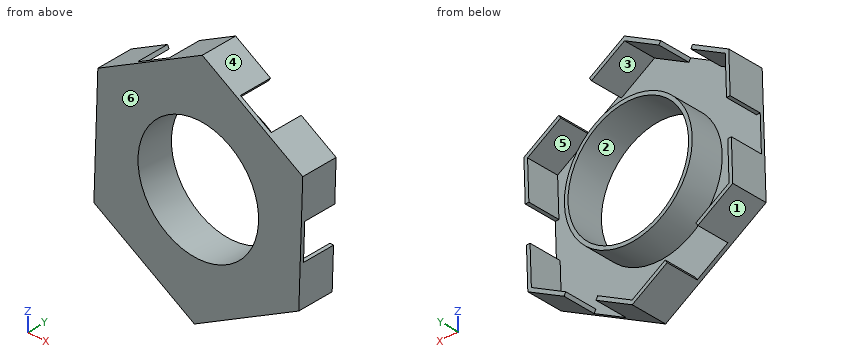
from build123d import *

# Parameters (mm, degrees)
SKETCH2_R           = 50
BOSS_EXTRUDE1_DEPTH = 30
SHELL1_T            = -3
CUT_EXTRUDE1_DEPTH  = 27


with BuildPart() as part:
    # Sketch2 → Boss-Extrude1 (new body)
    with BuildSketch(Plane(origin=(0, 0, 0), x_dir=(1, 0, 0), z_dir=(0, 1, 0))):
        Polygon((-83.314894361, -51.8841181), (3.275517147, -98.09487408), (86.590411508, -46.21075598), (83.314894361, 51.8841181), (-3.275517147, 98.09487408), (-86.590411508, 46.21075598), align=None)
        with Locations(Location((0, 0, 0), (0, 0, 270))):
            Circle(SKETCH2_R, mode=Mode.SUBTRACT)
    extrude(amount=BOSS_EXTRUDE1_DEPTH)

    # Shell1
    shell1_openings = [part.faces().sort_by_distance(p)[0] for p in [
        (-38.787596874, 30, 72.680784017),
    ]]
    offset(amount=SHELL1_T, openings=shell1_openings, kind=Kind.INTERSECTION)

    # Sketch8 → Cut-Extrude1 (cut)
    with BuildSketch(Plane(origin=(0, 30, 0), x_dir=(1, 0, 0), z_dir=(0, 1, 0))):
        Polygon((53.253129093, 67.9271981), (51.840669496, 65.280510003), (25.373788523, 79.405105982), (26.786248121, 82.051794079), align=None)
        Polygon((84.452062159, 17.828325695), (85.453243709, -12.154963576), (82.454914782, -12.255081731), (81.453733232, 17.72820754), align=None)
        Polygon((57.665814038, -64.223468384), (32.200114616, -80.082161676), (30.614245287, -77.535591734), (56.079944709, -61.676898442), align=None)
        Polygon((-26.786248121, -82.051794079), (-53.253129093, -67.9271981), (-51.840669496, -65.280510003), (-25.373788523, -79.405105982), align=None)
        Polygon((-84.452062159, -17.828325695), (-85.453243709, 12.154963576), (-82.454914782, 12.255081731), (-81.453733232, -17.72820754), align=None)
        Polygon((-57.665814038, 64.223468384), (-32.200114616, 80.082161676), (-30.614245287, 77.535591734), (-56.079944709, 61.676898442), align=None)
    extrude(amount=-CUT_EXTRUDE1_DEPTH, mode=Mode.SUBTRACT)


solid = part.part
Part model, mm, in its own coordinate system. Face numbers are marked on the shaded views. A direction names the side the tool comes from. Give positions to 0.01 mm unless a question says otherwise; leave off trailing zeros. Loops run counter-clockwise (first coordinate to the right, second up) from the corner with the lowest first, then second, coordinate; pieces in that order, holes last. Notation, with made-up numbers: M -16.5,-4 L 17.5,-4 A25 ccw 17.5,23 Z; hole C 58.5,53 d10. An arc over 180 degrees is marked long. Put each result on its own line as item: value. Start each with the question number.
1) Saw through at C-C (y = 18). State how many separate pieces and enclosed holes the cut face has, then the cut area to 3 significant figures.
2) 3-axis set-ups, long thin cutter, end or side, ignore diameter. For the marked faces 5 and 6: which of +Z, -Z, +X, -X, +Y, -Y reach the whole face in a straight line?
3) Saw through at B-B (z = 0). List the corners of the cut face in (x, y).
4) Flat gauge pins, fed straight in: pin 1 (4 mm diameter, centred on x = -51, z = -43, fed in from +Y); pin 2 (4 mm diameter, centred on y = 22.5, z = -48.5, fed in from +X); pin 3 (1 mm diameter, centred on y = 23.5, z = -6, fed in from +X). Where does each tip first touch, or does it go through?
5) Pull direction X, two halves, no side cores. Call the marked faces 1, 2, 3 and 4: +X half, -X half, draft (parallel to the pull), parting line (faces both ways), or undercut.
6) Saw through at A-A (x = -43). List the corners of the cut face in (y, z), then the cut area to 3 significant figures.
7) Probe probe 1 along X at (y, z) = (21, 0); probe 2 along X at (y, z) = (14, 30.5); probe 3 along X at (y, z) = (21, -40). List the from-to ranges inside material, lowest first.
8) Saw through at D-D (x = 9.5). List the corners of the cut face in (y, z), then the cut area to 3 significant figures.
Numbers:
1. separate pieces: 7
1. enclosed holes: 1
1. area: 2,170 mm^2
2. face 5: +Y
2. face 6: +Z, -Z, +X, -X, -Y
3. outline: M -85.05,0 L -50,0 L -50,30 L -53,30 L -53,3 L -85.05,3 Z; M 50,0 L 85.05,0 L 85.05,3 L 53,3 L 53,30 L 50,30 Z
4. pin 1: y = 3
4. pin 2: x = 83.49
4. pin 3: x = 52.71
5. face 1: -X half
5. face 2: undercut
5. face 3: undercut
5. face 4: +X half
6. outline: M 0,-73.36 L 3,-73.36 L 3,-30.98 L 30,-30.98 L 30,-25.51 L 0,-25.51 Z; M 0,25.51 L 30,25.51 L 30,30.98 L 3,30.98 L 3,73.4 L 0,73.4 Z
6. area: 583 mm^2
7. probe 1: -53 to -50, 50 to 53
7. probe 2: -84.03 to -81.03, -43.34 to -39.62, 39.62 to 43.34, 83.06 to 86.07
7. probe 3: -86.38 to -83.38, -34.77 to -30, 30 to 34.77, 80.71 to 83.71
8. outline: M 0,-91.28 L 30,-91.28 L 30,-87.88 L 3,-87.88 L 3,-52.14 L 30,-52.14 L 30,-49.09 L 0,-49.09 Z; M 0,49.09 L 30,49.09 L 30,52.14 L 3,52.14 L 3,90.68 L 30,90.68 L 30,94.22 L 0,94.22 Z
8. area: 614 mm^2
